Source: CAD feature listing. Evaluate the final solid. Frame: model axes, mm. A direction names the side the tool comes from. Coordinates: 2 decimals unless noted, no trailing zeros. Write each loop counter-clockwise with the first axis right and the second up, starting at its lowest first coordinate (ties: lowest second). Pieces come first, ordered by that corner, then holes. Notation, with made-up numbers: (-1, 42.25) -> (34, 42.25) arc R18 ccw to (34, 56.25) -> close; hole circle Ø2 at (39, -34.75). An arc over 180 degrees is marked (long way). Write item = value, one per line.
Autodesk Inventor part; units mm, degrees
ref_plane "YZ Plane" through (0, 0, 0) normal (1, 0, 0) x (0, 1, 0)
ref_plane "XZ Plane" through (0, 0, 0) normal (0, 1, 0) x (-1, 0, 0)
ref_plane "XY Plane" through (0, 0, 0) normal (0, 0, 1) x (1, 0, 0)
sketch "Sketch1" plane through (0, 0, 0) normal (0, 0, 1) x (1, 0, 0)
  line L0 (0, 0) -> (25.4, 0)
  line L1 (25.4, 0) -> (25.4, 50.8)
  line L2 (25.4, 50.8) -> (0, 50.8)
  line L3 (0, 50.8) -> (0, 0)
  dimension "d0" = 25.4
  dimension "d1" = 50.8
extrude "Extrusion1" add sketch "Sketch1" along normal blind 355.6
shell "Shell1" thickness 3.175 removed faces 2 at (16.9333, 16.9333, 0) at (8.4667, 33.8667, 355.6)
sketch "Sketch2" plane through (25.4, 0, 0) normal (1, 0, 0) x (0, 0, -1)
  line L0 (-355.6, 0) -> (-330.2, 0)
  line L1 (-330.2, 0) -> (-330.2, 25.4)
  line L2 (-330.2, 25.4) -> (-355.6, 25.4)
  line L3 (-355.6, 25.4) -> (-355.6, 0)
  line L4 (0, 0) -> (-25.4, 0)
  line L5 (-25.4, 0) -> (-25.4, 25.4)
  line L6 (-25.4, 25.4) -> (0, 25.4)
  line L7 (0, 25.4) -> (0, 0)
  dimension "d5" = 25.4
extrude "Extrusion2" cut sketch "Sketch2" against normal through all
sketch "Sketch3" plane through (25.4, 50.8, 355.6) normal (1, 0, 0) x (0, 0, -1)
  line L0 (330.2, -50.8) -> (330.2, -25.4)
  line L1 (25.4, -25.4) -> (25.4, -50.8)
  line L2 (330.2, -50.8) -> (25.4, -50.8)
  circle A0 centre (57.15, -38.1) radius 4.7625
  circle A1 centre (298.45, -38.1) radius 4.7625
  point P0 (355.6, -50.8)
  dimension "d8" = 9.525
  dimension "d9" = 31.75
  dimension "d10" = 12.7
  dimension "d11" = 12.7
  dimension "d12" = 31.75
extrude "Extrusion3" cut sketch "Sketch3" against normal through all
sketch "Sketch4" plane through (0, 50.8, 0) normal (0, 1, 0) x (1, 0, 0)
  line L0 (0, -355.6) -> (25.4, -355.6)
  line L1 (25.4, 0) -> (0, 0)
  line L2 (0, 0) -> (0, -355.6)
  circle A0 centre (12.7, -50.8) radius 3.175
  circle A1 centre (12.7, -304.8) radius 3.175
  line L3 (12.7, 0) -> (12.7, -50.8) construction
  line L4 (12.7, -50.8) -> (12.7, -304.8) construction
  line L5 (12.7, -304.8) -> (12.7, -355.6) construction
  dimension "d15" = 6.35
  dimension "d16" = 12.7
  dimension "d17" = 50.8
  dimension "d18" = 254
  dimension "d19" = 50.8
extrude "Extrusion4" cut sketch "Sketch4" against normal up to next
properties part number "Frame_MainHorizontalMount" material "Aluminum-6061"
1) Cut plane B-B, the plane y = 12.7. Output: boundary loops of the cut face in (x, z) (1 decimal), and give its area (3 significant figures).
Answer block:
outline = (0, 25.4) -> (3.2, 25.4) -> (3.2, 52.4) -> (0, 52.4) -> close; (0, 61.9) -> (3.2, 61.9) -> (3.2, 293.7) -> (0, 293.7) -> close; (0, 303.2) -> (3.2, 303.2) -> (3.2, 330.2) -> (0, 330.2) -> close; (22.2, 25.4) -> (25.4, 25.4) -> (25.4, 52.4) -> (22.2, 52.4) -> close; (22.2, 61.9) -> (25.4, 61.9) -> (25.4, 293.7) -> (22.2, 293.7) -> close; (22.2, 303.2) -> (25.4, 303.2) -> (25.4, 330.2) -> (22.2, 330.2) -> close
area = 1,810 mm2
2) Material intervals for probe 1 along Z at (x, y) = (12.7, 49.6) (3 decimals); probe 2 along Y at (x, z) = (10.25, 41.5) (3 decimals); probe 3 along X at (y, z) = (23.5, 58) (3 decimals), sorted ascending. Write a range as [from, to].
Answer block:
probe_1 = [0, 47.625], [53.975, 301.625], [307.975, 355.6]
probe_2 = [0, 3.175], [47.625, 50.8]
probe_3 = [0, 3.175], [22.225, 25.4]
3) Cut plane A-A, the plane z = 57.15. Output: boundary loops of the cut face in (x, y) (1 decimal), and give its area (3 significant figures).
Answer block:
outline = (0, 0) -> (25.4, 0) -> (25.4, 7.9) -> (22.2, 7.9) -> (22.2, 3.2) -> (3.2, 3.2) -> (3.2, 7.9) -> (0, 7.9) -> close; (0, 17.5) -> (3.2, 17.5) -> (3.2, 47.6) -> (22.2, 47.6) -> (22.2, 17.5) -> (25.4, 17.5) -> (25.4, 50.8) -> (0, 50.8) -> close
area = 383 mm2
4) First-contact query: pin 1 Ø1 at (x, z) = (1, 9) entering from -Y; pin 2 Ø5 at (x, z) = (12.7, 50.8) entering from +Y (3 decimals); pin 3 Ø10 at (x, y) = (15, 11.5) entering from -Z. Flat tips, straight axial feed; report the tip coordinate or a pass-through.
Answer block:
pin_1 = 25.4
pin_2 = 3.175
pin_3 = through
5) Pull-direction query (Z, two-part tool) for faces 5 (the flat face through (13, 2, 25.4)), 6 (the cylindrical face through (24, 11, 294)), 7 (the flat face through (25.4, 25, 175)), 8 (the cylindrical face through (12.29, 49.23, 301.65)); classes: +Z half, -Z half, draft (parallel to the pull), parting line (faces both ways), or undercut.
Answer block:
face_5 = -Z half
face_6 = undercut
face_7 = draft
face_8 = undercut
6) Cut plane C-C, the plane x = 12.7. Output: boundary loops of the cut face in (y, z) (3 decimals).
Answer block:
outline = (0, 25.4) -> (3.175, 25.4) -> (3.175, 330.2) -> (0, 330.2) -> close; (47.625, 0) -> (50.8, 0) -> (50.8, 47.625) -> (47.625, 47.625) -> close; (47.625, 53.975) -> (50.8, 53.975) -> (50.8, 301.625) -> (47.625, 301.625) -> close; (47.625, 307.975) -> (50.8, 307.975) -> (50.8, 355.6) -> (47.625, 355.6) -> close
7) Reachability of faces 1 (the flat face through (13, 2, 330.2)), 2 (the cylindrical face through (12.29, 49.23, 47.65)), 3 (the cylindrical face through (2, 11, 294)), 4 (the flat face through (22.225, 25, 175)) from +Z, -Z, +X, -X, +Y, -Y: full face, straight path, thin tool, end or side. Return the list, or none.
Answer block:
face_1 = +Z, +X, -X, -Y
face_2 = +Y
face_3 = +X, -X
face_4 = +Z, -Z
